Source: CAD feature listing. Evaluate the final solid. Frame: model axes, mm. Face numbers are marked on the shaded views. A direction names the side the tool comes from. Coordinates: 2 decimals unless noted, no trailing zeros. Order: outer loops, then holes, each group sorted by start corner. A loop starts at its lowest first (then second) coordinate and runs counter-clockwise, first axis right, second up.
Autodesk Inventor part; units mm, degrees
ref_plane "YZ Plane" through (0, 0, 0) normal (1, 0, 0) x (0, 1, 0)
ref_plane "XZ Plane" through (0, 0, 0) normal (0, 1, 0) x (-1, 0, 0)
ref_plane "XY Plane" through (0, 0, 0) normal (0, 0, 1) x (1, 0, 0)
sketch "スケッチ1" plane through (0, 0, 0) normal (0, 0, 1) x (1, 0, 0)
  line L0 (0, 16.25) -> (28.465632, 16.25) construction
  line L1 (28.465632, 16.25) -> (28.465632, -16.25) construction
  line L2 (28.465632, -16.25) -> (0, -16.25) construction
  line L3 (0, -16.25) -> (0, 16.25) construction
  line L4 (5, 23.25) -> (-5.158262, 23.25)
  line L5 (-5.158262, 23.25) -> (-34.5, 15.387905)
  line L6 (-34.5, 15.387905) -> (-34.5, -15.387905)
  line L7 (-34.5, -15.387905) -> (-5.158262, -23.25)
  line L8 (-5.158262, -23.25) -> (5, -23.25)
  line L9 (5, -23.25) -> (5, -16.3)
  line L10 (5, -16.3) -> (2.05, -16.3)
  arc A0 (-0.05, -16.3) -> (2.05, -16.3) centre (1, -16.3) ccw
  line L11 (-0.05, -16.3) -> (-0.05, 16.3)
  arc A1 (2.05, 16.3) -> (-0.05, 16.3) centre (1, 16.3) ccw
  line L12 (28.465632, 0) -> (0, 0) construction
  line L13 (2.05, 16.3) -> (5, 16.3)
  line L14 (5, 16.3) -> (5, 23.25)
  line L15 (28.515632, 16.3) -> (-0.05, 16.3) construction
  line L16 (-0.05, 16.3) -> (-0.05, -16.3) construction
  line L17 (-0.05, -16.3) -> (28.515632, -16.3) construction
  line L18 (28.515632, -16.3) -> (28.515632, 16.3) construction
  circle A2 centre (-4.5, 18.25) radius 1.2
  circle A3 centre (-4.5, -18.25) radius 1.2
  line L19 (0, 0) -> (28.465632, 0) construction
  line L20 (2.5, 16.25) -> (2.5, -16.25) construction
  circle A4 centre (-4.5, 18.25) radius 5 construction
  line L21 (-6.087713, 15.5) -> (-7.675426, 18.25)
  line L22 (-7.675426, 18.25) -> (-6.087713, 21)
  line L23 (-6.087713, 21) -> (-2.912287, 21)
  line L24 (-2.912287, 21) -> (-1.324574, 18.25)
  line L25 (-1.324574, 18.25) -> (-2.912287, 15.5)
  line L26 (-2.912287, 15.5) -> (-6.087713, 15.5)
  point P0 (-34.5, 0)
  point P1 (-0.05, 0)
  dimension "d98" = 32.5
  dimension "d100" = 0.05
  dimension "d101" = 1.05
  dimension "d102" = 5
  dimension "d104" = 2.4
  dimension "d106" = 2.5
  dimension "d107" = 7
  dimension "d108" = 18.25
  dimension "d109" = 5
  dimension "d110" = 30
  dimension "d111" = 165
  dimension "d130" = 5.5
extrude "押し出し1" add sketch "スケッチ1" along normal blind 5 contours L14 L13 A1 L11 A0 L10 L9 L8 L7 L6 L5 L4 | L21 L22 L23 L24 L25 L26
sketch "スケッチ6" plane through (0, 0, 0) normal (0, 0, -1) x (-1, 0, 0)
  line L0 (34.5, -15.387905) -> (5.158262, -23.25)
  line L1 (34.5, 15.387905) -> (34.5, -15.387905)
  line L2 (5.158262, 23.25) -> (34.5, 15.387905)
  line L3 (8.5, 17.178203) -> (8.5, -17.178203)
  line L4 (8.5, -17.178203) -> (29.5, -11.55127)
  line L5 (29.5, -11.55127) -> (29.5, 11.55127)
  line L6 (29.5, 11.55127) -> (8.5, 17.178203)
  circle A0 centre (4.5, 18.25) radius 1.2
  point P0 (0, 0)
  dimension "d113" = 5
  dimension "d114" = 5
  dimension "d115" = 5
  dimension "d133" = 4
extrude "押し出し4" cut sketch "スケッチ6" against normal blind 4 contours L6 L5 L4 L3
fillet "フィレット2" radius 1.05 4 edges at (-8.5, 17.1782, 2) (-8.5, -17.1782, 2) (-29.5, 11.5513, 2) (-29.5, -11.5513, 2)
sketch "スケッチ7" plane through (0, 0, 0) normal (0, 0, -1) x (-1, 0, 0)
  circle A0 centre (4.5, -18.25) radius 1.2
  circle A1 centre (4.5, 18.25) radius 1.2
  line L0 (2.912287, 15.5) -> (1.324574, 18.25)
  line L1 (1.324574, 18.25) -> (2.912287, 21)
  line L2 (2.912287, 21) -> (6.087713, 21)
  line L3 (6.087713, 21) -> (7.675426, 18.25)
  line L4 (7.675426, 18.25) -> (6.087713, 15.5)
  line L5 (6.087713, 15.5) -> (2.912287, 15.5)
  line L6 (7.6812, 18.25) -> (6.0906, 21.005)
  line L7 (6.0906, 21.005) -> (2.9094, 21.005)
  line L8 (2.9094, 21.005) -> (1.3188, 18.25)
  line L9 (1.3188, 18.25) -> (2.9094, 15.495)
  line L10 (2.9094, 15.495) -> (6.0906, 15.495)
  line L11 (6.0906, 15.495) -> (7.6812, 18.25)
  circle A2 centre (6.6312, 18.25) radius 1.05
  circle A3 centre (5.5656, 20.095673) radius 1.05
  circle A4 centre (3.4344, 20.095673) radius 1.05
  circle A5 centre (2.3688, 18.25) radius 1.05
  circle A6 centre (3.4344, 16.404327) radius 1.05
  circle A7 centre (5.5656, 16.404327) radius 1.05
  line L12 (7.6812, -18.25) -> (6.0906, -21.005)
  line L13 (6.0906, -21.005) -> (2.9094, -21.005)
  line L14 (2.9094, -21.005) -> (1.3188, -18.25)
  line L15 (1.3188, -18.25) -> (2.9094, -15.495)
  line L16 (2.9094, -15.495) -> (6.0906, -15.495)
  line L17 (6.0906, -15.495) -> (7.6812, -18.25)
  circle A8 centre (6.6312, -18.25) radius 1.05
  circle A9 centre (5.5656, -16.404327) radius 1.05
  circle A10 centre (3.4344, -16.404327) radius 1.05
  circle A11 centre (2.3688, -18.25) radius 1.05
  circle A12 centre (3.4344, -20.095673) radius 1.05
  circle A13 centre (5.5656, -20.095673) radius 1.05
  point P0 (0, 0)
  point P1 (6.0906, 21.005)
  point P2 (2.9094, 21.005)
  point P3 (1.3188, 18.25)
  point P4 (2.9094, 15.495)
  point P5 (6.0906, 15.495)
  point P6 (2.9094, -15.495)
  point P7 (2.9094, -21.005)
  point P8 (6.0906, -21.005)
  dimension "d121" = 2.1
  dimension "d119" = 5.5
  dimension "d120" = 0.005
  dimension "d124" = 360
  dimension "d128" = 360
sketch "スケッチ7 outline for 押し出し5" plane through (0, 0, 0) normal (0, 0, -1) x (-1, 0, 0)
  arc A0 (6.6156, 20.095673) -> (5.0406, 21.005) centre (5.5656, 20.095673) ccw
  line L0 (5.0406, 21.005) -> (3.9594, 21.005)
  arc A1 (3.9594, 21.005) -> (2.3844, 20.095673) centre (3.4344, 20.095673) ccw
  line L1 (2.3844, 20.095673) -> (1.8438, 19.159327)
  arc A2 (1.8438, 19.159327) -> (1.8438, 17.340673) centre (2.3688, 18.25) ccw
  line L2 (1.8438, 17.340673) -> (2.3844, 16.404327)
  arc A3 (2.3844, 16.404327) -> (3.9594, 15.495) centre (3.4344, 16.404327) ccw
  line L3 (3.9594, 15.495) -> (5.0406, 15.495)
  arc A4 (5.0406, 15.495) -> (6.6156, 16.404327) centre (5.5656, 16.404327) ccw
  line L4 (6.6156, 16.404327) -> (7.1562, 17.340673)
  arc A5 (7.1562, 17.340673) -> (7.1562, 19.159327) centre (6.6312, 18.25) ccw
  line L5 (7.1562, 19.159327) -> (6.6156, 20.095673)
  arc A6 (6.6156, -16.404327) -> (5.0406, -15.495) centre (5.5656, -16.404327) ccw
  line L6 (3.9594, -15.495) -> (5.0406, -15.495)
  arc A7 (3.9594, -15.495) -> (2.3844, -16.404327) centre (3.4344, -16.404327) ccw
  line L7 (1.8438, -17.340673) -> (2.3844, -16.404327)
  arc A8 (1.8438, -17.340673) -> (1.8438, -19.159327) centre (2.3688, -18.25) ccw
  line L8 (2.3844, -20.095673) -> (1.8438, -19.159327)
  arc A9 (2.3844, -20.095673) -> (3.9594, -21.005) centre (3.4344, -20.095673) ccw
  line L9 (5.0406, -21.005) -> (3.9594, -21.005)
  arc A10 (5.0406, -21.005) -> (6.6156, -20.095673) centre (5.5656, -20.095673) ccw
  line L10 (7.1562, -19.159327) -> (6.6156, -20.095673)
  arc A11 (7.1562, -19.159327) -> (7.1562, -17.340673) centre (6.6312, -18.25) ccw
  line L11 (6.6156, -16.404327) -> (7.1562, -17.340673)
  arc A12 (5.644781, -17.890171) -> (5.384012, -17.438505) centre (4.5, -18.25) ccw
  arc A13 (5.644781, -17.890171) -> (5.644781, -18.609829) centre (6.6312, -18.25) ccw
  arc A14 (5.384012, -19.061495) -> (5.644781, -18.609829) centre (4.5, -18.25) ccw
  arc A15 (5.384012, -19.061495) -> (4.760769, -19.421324) centre (5.5656, -20.095673) ccw
  arc A16 (4.239231, -19.421324) -> (4.760769, -19.421324) centre (4.5, -18.25) ccw
  arc A17 (4.239231, -19.421324) -> (3.615988, -19.061495) centre (3.4344, -20.095673) ccw
  arc A18 (3.355219, -18.609829) -> (3.615988, -19.061495) centre (4.5, -18.25) ccw
  arc A19 (3.355219, -18.609829) -> (3.355219, -17.890171) centre (2.3688, -18.25) ccw
  arc A20 (3.615988, -17.438505) -> (3.355219, -17.890171) centre (4.5, -18.25) ccw
  arc A21 (3.615988, -17.438505) -> (4.239231, -17.078676) centre (3.4344, -16.404327) ccw
  arc A22 (4.760769, -17.078676) -> (4.239231, -17.078676) centre (4.5, -18.25) ccw
  arc A23 (4.760769, -17.078676) -> (5.384012, -17.438505) centre (5.5656, -16.404327) ccw
extrude "押し出し5" cut sketch "スケッチ7 outline for 押し出し5" against normal blind 2
equation "\"d114\" = d113"
equation "\"d115\" = d113"
properties part number "胴体_サブフレーム_1_7" material "アセタール樹脂、黒"
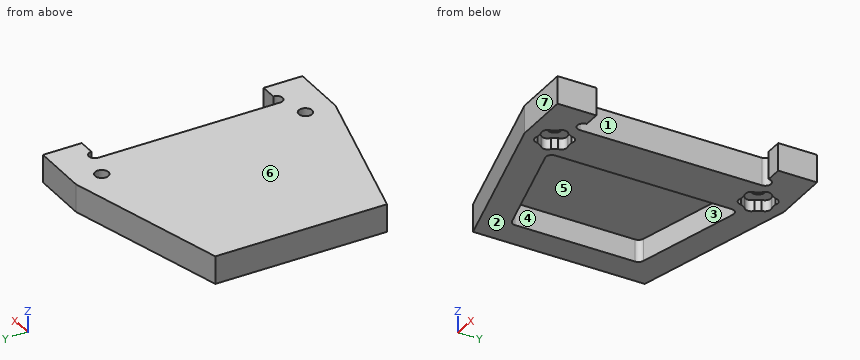
1. Section query A-A on x = -4.5. Return loops of the section in (y, z) (3 decimals), plus the area to 3 significant figures.
Findings:
outline: (-23.25, 0) - (-21.005, 0) - (-21.005, 2) - (-19.45, 2) - (-19.45, 5) - (-23.25, 5) - close; (-17.05, 2) - (-15.495, 2) - (-15.495, 0) - (15.495, 0) - (15.495, 2) - (17.05, 2) - (17.05, 5) - (-17.05, 5) - close; (19.45, 2) - (21.005, 2) - (21.005, 0) - (23.25, 0) - (23.25, 5) - (19.45, 5) - close
area: 196 mm2
2. Section query B-B on z = 3.3. Return loops of the section in (x, y), plus the area to 3 significant figures.
Findings:
outline: (-34.5, -15.39) - (-5.16, -23.25) - (5, -23.25) - (5, -16.3) - (2.05, -16.3) arc R1.05 cw to (-0.05, -16.3) - (-0.05, 16.3) arc R1.05 cw to (2.05, 16.3) - (5, 16.3) - (5, 23.25) - (-5.16, 23.25) - (-34.5, 15.39) - close; hole (-29.5, -10.75) arc R1.05 ccw to (-28.72, -11.76) - (-9.82, -16.82) arc R1.05 ccw to (-8.5, -15.81) - (-8.5, 15.81) arc R1.05 ccw to (-9.82, 16.82) - (-28.72, 11.76) arc R1.05 ccw to (-29.5, 10.75) - close; hole circle Ø2.4 at (-4.5, -18.25); hole circle Ø2.4 at (-4.5, 18.25)
area: 827 mm2
3. Section query D-D on y = 18.25. Return loops of the section in (x, z).
Findings:
outline: (-23.82, 0) - (-7.68, 0) - (-7.68, 2) - (-5.7, 2) - (-5.7, 5) - (-23.82, 5) - close; (-3.3, 2) - (-1.32, 2) - (-1.32, 0) - (5, 0) - (5, 5) - (-3.3, 5) - close
4. Pin query (flat end, axial travel): P1, Ø1, axis at y = 8.5, z = 2.5, coming from the +X side; P2, Ø3, axis at x = -4.5, y = -18.25, coming from the -Z side. Return the tip coordinate at first contact, or that it passes through.
Findings:
P1: stops at x = -0.05
P2: stops at z = 2
5. Access query for the marked faces 1, 2 and 3. Directions: +Z, -Z, +X, -X, +Y, -Y. A direction counts if a zero-diameter tool reaches every point of the face in a straight line with its end or side. Return the directions, or none.
Findings:
face 1: +Z, -Z, +X
face 2: -Z, +X, -X, +Y, -Y
face 3: -Z
6. Draft query along Y for the marked faces 4, 5, 6 and 7. Return one class per face: released by +Y, released by -Y, zero draft, split by the parting line, or undercut.
Findings:
face 4: undercut
face 5: undercut
face 6: zero draft
face 7: released by -Y
7. Section query C-C on x = 1. Return loops of the section in (y, z).
Findings:
outline: (-23.25, 0) - (-17.35, 0) - (-17.35, 5) - (-23.25, 5) - close; (17.35, 0) - (23.25, 0) - (23.25, 5) - (17.35, 5) - close
8. Ray query, line 1 (Y direction, x = -4.5, z = 3.1); line 2 (X direction, y = 0, z = 0.4); line 3 (Y direction, x = -1.5, z = 0.55). Return the intervals inside material, ascending.
Findings:
line 1: y = -23.25 to -19.45, -17.05 to 17.05, 19.45 to 23.25
line 2: x = -34.5 to -29.5, -8.5 to -0.05
line 3: y = -23.25 to -18.84, -17.66 to 17.66, 18.84 to 23.25
